Model file for the job. Use its own axes, mm. Face numbers are marked on the shaded views. A direction names the side the tool comes from. Round coordinates to 2 decimals unless told otherwise and drop trailing zeros. Loops run counter-clockwise (first coordinate to the right, second up) from the corner with the lowest first, then second, coordinate; pieces in that order, holes last. Notation, with made-up numbers: (49, 88) - (96, 88) arc R19 cw to (96, 108) - close; hole circle Ø2 at (-4.75, 46). An arc over 180 degrees is marked (long way). Answer as a JSON object with one key per item and string values.
from build123d import *

# Parameters (mm, degrees)
EXTRUDE_1_DEPTH      = 40
EXTRUDE_1_DEPTH_BACK = 5
SKETCH_2_W           = 36
SKETCH_2_H           = 37
CUT_EXTRUDE_1_DEPTH  = 50
SKETCH_5_W           = 36
SKETCH_5_H           = 5
CUT_EXTRUDE_4_DEPTH  = 43
SKETCH_9_R           = 1.025
CUT_EXTRUDE_5_DEPTH  = 45.5
SKETCH_10_W          = 3
SKETCH_10_H          = 8
EXTRUDE_4_DEPTH      = 10
SKETCH_12_R          = 1.05
CUT_EXTRUDE_6_DEPTH  = 10
FILLET_4_R           = 2
FILLET_5_R           = 2
FILLET_6_R           = 2
FILLET_7_R           = 2


with BuildPart() as part:
    # 草圖1 → 填料-伸長1 (new body, two sides)
    with BuildSketch(Plane.XY) as extrude_1_sk:
        Polygon((-14.545454545, -28.090909091), (-15.545454545, -28.090909091), (-15.545454545, 16.909090909), (-14.545454545, 16.909090909), (25.454545455, 16.909090909), (26.454545455, 16.909090909), (26.454545455, -28.090909091), (25.454545455, -28.090909091), align=None)
    extrude(amount=EXTRUDE_1_DEPTH)
    extrude(extrude_1_sk.sketch, amount=-EXTRUDE_1_DEPTH_BACK)

    # 草圖2 → 除料-伸長1 (cut)
    with BuildSketch(Plane(origin=(0, 16.909090909, 0), x_dir=(1, 0, 0), z_dir=(0, 1, 0))):
        with Locations((5.454545455, -21.5)):
            Rectangle(SKETCH_2_W, SKETCH_2_H)
    extrude(amount=-CUT_EXTRUDE_1_DEPTH, mode=Mode.SUBTRACT)

    # 草圖5 → 除料-伸長4 (cut)
    with BuildSketch(Plane(origin=(0, 16.909090909, 0), x_dir=(1, 0, 0), z_dir=(0, 1, 0))):
        with Locations((5.454545455, -0.5)):
            Rectangle(SKETCH_5_W, SKETCH_5_H)
    extrude(amount=-CUT_EXTRUDE_4_DEPTH, mode=Mode.SUBTRACT)

    # 草圖9 → 除料-伸長5 (cut)
    with BuildSketch(Plane.ZY.offset(15.545454545)):
        with Locations((37, -25.090909091)):
            Circle(SKETCH_9_R)
        with Locations((37, 13.909090909)):
            Circle(SKETCH_9_R)
    extrude(amount=-CUT_EXTRUDE_5_DEPTH, mode=Mode.SUBTRACT)

    # 草圖10 → 填料-伸長4 (add)
    with BuildSketch(Plane(origin=(0, 16.909090909, 0), x_dir=(1, 0, 0), z_dir=(0, 1, 0))):
        with Locations((-14.045454545, -17.5)):
            Rectangle(SKETCH_10_W, SKETCH_10_H)
        with Locations((24.954545455, -17.5)):
            Rectangle(SKETCH_10_W, SKETCH_10_H)
    extrude(amount=EXTRUDE_4_DEPTH)

    # 草圖12 → 除料-伸長6 (cut)
    with BuildSketch(Plane(origin=(0, 0, 13.5), x_dir=(-1, 0, 0), z_dir=(0, 0, -1))):
        with Locations((-24.954545455, 21.909090909)):
            Circle(SKETCH_12_R)
        with Locations((14.045454545, 21.909090909)):
            Circle(SKETCH_12_R)
    extrude(amount=-CUT_EXTRUDE_6_DEPTH, mode=Mode.SUBTRACT)

    # 圓角4
    fillet_4_edges = [part.edges().sort_by_distance(p)[0] for p in [
        (26.454545455, -5.590909091, -5),
    ]]
    fillet(fillet_4_edges, radius=FILLET_4_R)

    # 圓角5
    fillet_5_edges = [part.edges().sort_by_distance(p)[0] for p in [
        (-15.545454545, -5.590909091, -5),
    ]]
    fillet(fillet_5_edges, radius=FILLET_5_R)

    # 圓角6
    fillet_6_edges = [part.edges().sort_by_distance(p)[0] for p in [
        (26.454545455, -5.590909091, 40),
    ]]
    fillet(fillet_6_edges, radius=FILLET_6_R)

    # 圓角7
    fillet_7_edges = [part.edges().sort_by_distance(p)[0] for p in [
        (-15.545454545, -5.590909091, 40),
    ]]
    fillet(fillet_7_edges, radius=FILLET_7_R)


solid = part.part
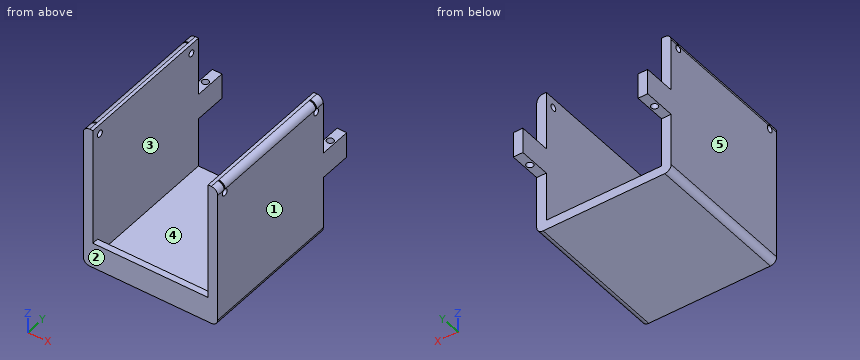
1) Probe probe 1 along X at (y, z) = (8, 1.5); probe 2 along Z at (x, y) = (8, -25); probe 3 along Y at (x, z) = (22.5, -1.5). List the from-to ranges inside material, lowest first.
Values follow:
{"probe 1": "-15.55 to -12.55, 23.45 to 26.45", "probe 2": "-5 to -2", "probe 3": "-28.09 to -26.09"}
2) Slice it at C-C on z = 0. List the corners of the cut face in (x, y), then the cut area to 3 significant figures.
Values follow:
{"outline": "(-15.55, -28.09) - (26.45, -28.09) - (26.45, 16.91) - (23.45, 16.91) - (23.45, -26.09) - (-12.55, -26.09) - (-12.55, 16.91) - (-15.55, 16.91) - close", "area": "342 mm²"}
3) Slice it at D-D on y = -13. List the corners of the cut face in (x, z).
Values follow:
{"outline": "(-15.55, -3) arc R2 ccw to (-13.55, -5) - (24.45, -5) arc R2 ccw to (26.45, -3) - (26.45, 38) arc R2 ccw to (24.45, 40) - (23.45, 40) - (23.45, -2) - (-12.55, -2) - (-12.55, 40) - (-13.55, 40) arc R2 ccw to (-15.55, 38) - close"}
4) Slice it at B-B on z = 7. List the corners of the cut face in (x, y).
Values follow:
{"outline": "(-15.55, -28.09) - (-12.55, -28.09) - (-12.55, 16.91) - (-15.55, 16.91) - close; (23.45, -28.09) - (26.45, -28.09) - (26.45, 16.91) - (23.45, 16.91) - close"}
5) Two-plate mould, pull along X, no slides. Class the marked faces 1, 2 and 3: pulls with the +X half, pulls with the -X half, needs draft (parallel to the pull), parting line crosses it, or undercut.
Values follow:
{"face 1": "pulls with the +X half", "face 2": "needs draft", "face 3": "undercut"}
6) Slice it at A-A on z = 37. List the corners of the cut face in (x, y), then the cut area to 3 significant figures.
Values follow:
{"outline": "(-15.55, -28.09) - (-12.55, -28.09) - (-12.55, -26.12) - (-15.55, -26.12) - close; (-15.55, -24.07) - (-12.55, -24.07) - (-12.55, 12.88) - (-15.55, 12.88) - close; (-15.55, 14.93) - (-12.55, 14.93) - (-12.55, 16.91) - (-15.55, 16.91) - close; (23.45, -28.09) - (26.45, -28.09) - (26.45, -26.12) - (23.45, -26.12) - close; (23.45, -24.07) - (26.45, -24.07) - (26.45, 12.88) - (23.45, 12.88) - close; (23.45, 14.93) - (26.45, 14.93) - (26.45, 16.91) - (23.45, 16.91) - close", "area": "245 mm²"}
7) Tool access for the marked faces 4 and 5: list every direction of +Z, -Z, +X, -X, +Y, -Y with a clear straight run to the whole face (end or side of a thin tool).
Values follow:
{"face 4": "+Z, +Y", "face 5": "+Z, -Z, -X, +Y, -Y"}
8) Drop flat-ended pins along their axis: P1, Ø3.5, axis at x = 25, y = 23, coming from the +Z side; P2, Ø0.9, axis at x = 25, y = 20.5, coming from the -Z side; P3, Ø0.6, axis at x = 14, y = -27, coming from the +Z side; P4, Ø2.5, axis at y = -25.09, z = 37, coming from the +X side. Give the stop position or say it passes through.
Values follow:
{"P1": "z = 21.5", "P2": "z = 13.5", "P3": "z = 3", "P4": "x = 26.45"}
